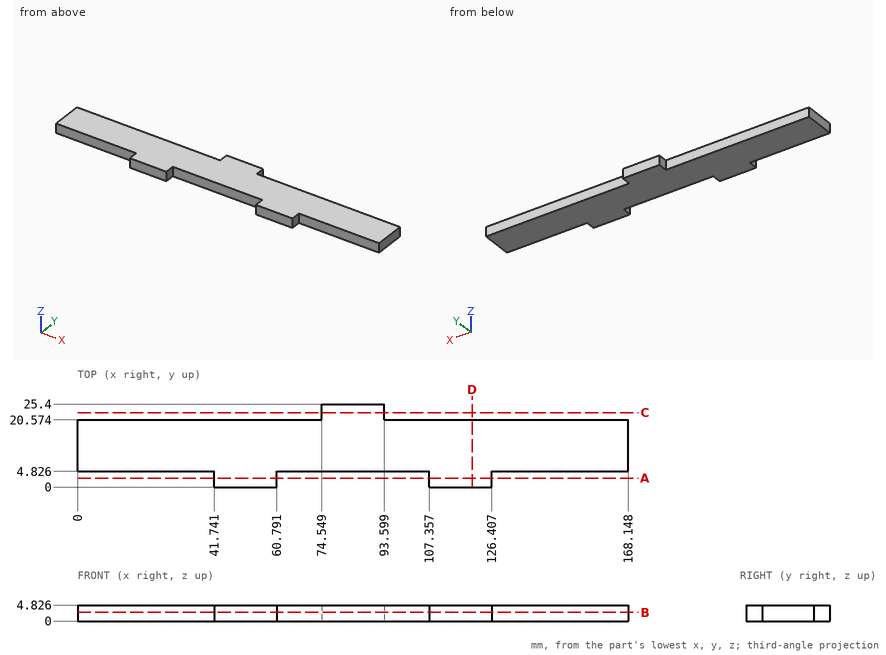
For this review, use the dimensioned drawing (mm, ordinates from the lowest corner) and the shaded views. Round coordinates to 2 decimals unless told otherwise and drop trailing zeros. Write each loop counter-clockwise with the first axis right and the second up, starting at its lowest first coordinate (ties: lowest second). Pieces come first, ordered by that corner, then holes. Notation, with made-up numbers: (19, 26.25) -> (23, 26.25) arc R33 ccw to (23, 63.25) -> close; hole circle Ø10 at (-29, -6). An arc over 180 degrees is marked (long way). Use one line per item in the form item = value.
Q1. Clearance check with flat-ended pins moving along their axes: pin 1 Ø2.5 at (x, z) = (77, 3) entering from -Y; pin 2 Ø1.4 at (y, z) = (3.5, 3) entering from +X; pin 3 Ø2.5 at (y, z) = (23.5, 3.5) entering from +X. State where each tip first meets the part, or that it passes through.
Resolved:
pin_1 = 4.83
pin_2 = 126.41
pin_3 = 93.6
Q2. To check wall thickness, follow probe 1 along X at (y, z) = (2.25, 2.25); probe 2 along X at (y, z) = (23.5, 3.05); probe 3 along Y at (x, z) = (141, 1.4). State the ranges of each line that lie inside material, in increasing order. Write a range as from..to.
Resolved:
probe_1 = 41.74..60.79, 107.36..126.41
probe_2 = 74.55..93.6
probe_3 = 4.83..20.57
Q3. Consider section A-A (y = 2.75). State the section outline as (x, z) points.
Resolved:
outline = (41.74, 0) -> (60.79, 0) -> (60.79, 4.83) -> (41.74, 4.83) -> close; (107.36, 0) -> (126.41, 0) -> (126.41, 4.83) -> (107.36, 4.83) -> close
Q4. Consider section C-C (y = 22.75). State the section outline as (x, z) points.
Resolved:
outline = (74.55, 0) -> (93.6, 0) -> (93.6, 4.83) -> (74.55, 4.83) -> close
Q5. Consider section B-B (z = 2.6). State the section outline as (x, y) points, then the cut area to 3 significant figures.
Resolved:
outline = (0, 4.83) -> (41.74, 4.83) -> (41.74, 0) -> (60.79, 0) -> (60.79, 4.83) -> (107.36, 4.83) -> (107.36, 0) -> (126.41, 0) -> (126.41, 4.83) -> (168.15, 4.83) -> (168.15, 20.57) -> (93.6, 20.57) -> (93.6, 25.4) -> (74.55, 25.4) -> (74.55, 20.57) -> (0, 20.57) -> close
area = 2,920 mm²
Q6. Consider section D-D (x = 120.5). State the section outline as (y, z) points.
Resolved:
outline = (0, 0) -> (20.57, 0) -> (20.57, 4.83) -> (0, 4.83) -> close
